The model under review builds one solid part; all positions refer to its coordinate system, in mm. A direction names the side the tool comes from. Round coordinates to 2 decimals unless told otherwise and drop trailing zeros.
```python
from build123d import *

# Parameters (mm, degrees)
SKETCH4_R          = 2.5
CUT_EXTRUDE1_DEPTH = 10


with BuildPart() as part:
    # Sketch1 → Revolve1 (revolve)
    with BuildSketch(Plane.XY, mode=Mode.PRIVATE) as revolve1_sk:
        with BuildLine():
            Line((0, 0), (0, 320))
            Line((0, 320), (0, 331.054218753))
            Line((0, 331.054218753), (13, 331.054218753))
            Line((13, 331.054218753), (13, 321.576985446))
            Line((13, 321.576985446), (15.433464657, 320))
            Line((15.433464657, 320), (13, 320))
            add(Edge.make_bspline(
                [(13, 320), (11.878091836, 283.27832547), (50.721966152, 265.475319412), (52.567488524, 229.937180409)],
                knots=[0, 0, 0, 0, 1, 1, 1, 1], degree=3))
            Line((52.567488524, 229.937180409), (52.567488524, 132.323370386))
            add(Edge.make_bspline(
                [(52.567488524, 132.323370386), (55.245477634, 101.880070943), (44.248099594, 56.601355946), (64.997390408, 10.768245845), (44.287893313, 0)],
                knots=[0, 0, 0, 0, 0.662490956, 1, 1, 1, 1], degree=3))
            Line((44.287893313, 0), (0, 0))
        make_face()
    revolve(revolve1_sk.sketch.rotate(Axis((0, 0, 0), (0, 1, 0)), 90), axis=Axis((0, 0, 0), (0, 1, 0)))

    # Sketch2 → Revolve2 (revolve)
    with BuildSketch(Plane.XY, mode=Mode.PRIVATE) as revolve2_sk:
        with BuildLine():
            Line((4.280433448, 347.757883162), (0, 347.757883162))
            Line((0, 347.757883162), (0, 320))
            Line((0, 320), (15.433464657, 320))
            ThreePointArc((15.433464657, 320), (9.079705094, 333.566647373), (4.280433448, 347.757883162))
        make_face()
    revolve(revolve2_sk.sketch.rotate(Axis((0, 347.757883162, 0), (0, -1, 0)), 180), axis=Axis((0, 347.757883162, 0), (0, -1, 0)))

    # Sketch3 → Cut-Revolve1 (revolve, cut)
    with BuildSketch(Plane.XY, mode=Mode.PRIVATE) as cut_revolve1_sk:
        with BuildLine():
            Line((9.919015749, 331.054218753), (13, 331.054218753))
            Line((13, 331.054218753), (13, 324.743018777))
            ThreePointArc((13, 324.743018777), (11.37547872, 327.857597644), (9.919015749, 331.054218753))
        make_face()
    revolve(cut_revolve1_sk.sketch.rotate(Axis((0, 331.054218753, 0), (0, 1, 0)), 180), axis=Axis((0, 331.054218753, 0), (0, 1, 0)), mode=Mode.SUBTRACT)

    # Sketch4 → Cut-Extrude1 (cut)
    with BuildSketch(Plane(origin=(0, 347.757883162, 0), x_dir=(1, 0, 0), z_dir=(0, 1, 0))):
        with Locations(Location((0, 0, 0), (0, 0, 180))):
            Circle(SKETCH4_R)
    extrude(amount=-CUT_EXTRUDE1_DEPTH, mode=Mode.SUBTRACT)


solid = part.part
```
(1) For faces 1 (the cylindrical face through (-2.311, 180.447, 52.517)), 2 (the flat face through (-2, 347.758, 2)), 3 (the flat face through (11.4, 320, 6.9)), list the 3-axis set-ups (+Z, -Z, +X, -X, +Y, -Y) from which the entire face can be reached by the end or side of a thin tool; tool diameter is ignored.
Data:
face 1: +Y
face 2: +Z, -Z, +X, -X, +Y
face 3: none
(2) Insertion check: pin 1 (6 mm diameter, centred on y = 277.5, z = 19.5, fed in from +X); pin 2 (4.5 mm diameter, centred on x = 0, z = 0, fed in from +Y); pin 3 (5 mm diameter, centred on x = -2, z = 12, fed in from +Y). Each pin has a flat end and moves straight along its axis. Give the tip position at first contact, or say it passes through.
Data:
pin 1: stops at x = 25.76
pin 2: stops at y = 337.76
pin 3: stops at y = 332.13
(3) To check wall thickness, follow probe 1 along Z at (x, y) = (0, 340); probe 2 along Z at (x, y) = (0, 344); probe 3 along Z at (x, y) = (-11.5, 28). State the ranges of each line that lie inside material, in increasing order.
Data:
probe 1: z = -6.68 to -2.5, 2.5 to 6.68
probe 2: z = -5.38 to -2.5, 2.5 to 5.38
probe 3: z = -56.61 to 56.61
